```python
from build123d import *

# Parameters (mm, degrees)
F0_W            = 19
F0_H            = 19
F1_DEPTH        = 1
F2_W            = 17
F2_H            = 17
F3_DEPTH        = 4
F4_T            = 1
F4_T3_DEPTH     = 19
F4_T5_DEPTH     = 19
F6_DEPTH        = 2
F6_COPIES_COUNT = 4
F8_R            = 1
F9_SIZE         = 0.5


# Not quite as in the source:
# - a pattern or mirror of a feature is missing from the dataset's text; its kind, count and spacing are read off the source's solid
# - a shell that OpenCascade refuses in one call is made with other operations: the cavity is built on its own and cut out


with BuildPart() as f1:
    # F0 (on Top) → F1 (new body)
    with BuildSketch(Plane.XY):
        Rectangle(F0_W, F0_H)
    extrude(amount=F1_DEPTH)

    # F2 (on face) → F3 (join)
    with BuildSketch(Plane.XY.offset(1)):
        Rectangle(F2_W, F2_H)
    extrude(amount=F3_DEPTH)

    # F4: shell of thickness 1, made by hand


with BuildPart() as f4_core1:
    # F4_t2: copy of F1
    add(f1.part)

    # the walls: a layer under each face that stays
    f4_faces = [f4_core1.faces().sort_by_distance(p)[0] for p in [
        (0, -9.5, 0.5),
        (-9.5, 0, 0.5),
        (9.5, 0, 0.5),
        (0, 0, 0),
        (-8.8666666667, -8.8666666667, 1),
        (0, 9.5, 0.5),
        (8.5, 0, 3),
        (0, 8.5, 3),
        (-8.5, 0, 3),
        (0, -8.5, 3),
    ]]
    thicken(f4_faces, amount=-F4_T, mode=Mode.SUBTRACT)

    # F4_s4 → F4_t3 (cut)
    with BuildSketch(Plane.XZ.offset(-9.5)):
        Polygon((8.51, 1.01), (8.5, 0), (7.5, 0), (7.5, 1), align=None)
        Polygon((-8.51, 1.01), (-8.5, 0), (-7.5, 0), (-7.5, 1), align=None)
    extrude(amount=F4_T3_DEPTH, mode=Mode.SUBTRACT)

    # F4_s6 → F4_t5 (cut)
    with BuildSketch(Plane.YZ.offset(-9.5)):
        Polygon((8.51, 1.01), (8.5, 0), (7.5, 0), (7.5, 1), align=None)
        Polygon((-8.51, 1.01), (-8.5, 0), (-7.5, 0), (-7.5, 1), align=None)
    extrude(amount=F4_T5_DEPTH, mode=Mode.SUBTRACT)


with BuildPart() as f1_1:
    add(f1.part)

    # what is left inside the walls is the cavity
    f4_cavity = [f4_core1.part.solids().sort_by_distance(p)[0] for p in [
        (0, -2.5, 1.01),
    ]]
    add(f4_cavity, mode=Mode.SUBTRACT)

    # F5 (on face) → F6 (cut)
    with BuildSketch(Plane.XZ.offset(8.5)):
        with BuildLine():
            Line((5.5, 5), (-5.5, 5))
            ThreePointArc((-5.5, 5), (0, 2.8094750193), (5.5, 5))
        make_face()
    f6 = extrude(amount=-F6_DEPTH, mode=Mode.SUBTRACT)

    # F6_copies: F6 ×4 about axis
    f6_copies_axis = Axis((0, 0, 0), (0, 0, 1))
    for i in range(1, F6_COPIES_COUNT):
        add(f6.rotate(f6_copies_axis, i * 360 / F6_COPIES_COUNT), mode=Mode.SUBTRACT)

    # F8
    f8_edges = [f1_1.edges().sort_by_distance(p)[0] for p in [
        (-8.5, -8.5, 3),
        (-9.5, -9.5, 0.5),
        (8.5, -8.5, 3),
        (9.5, -9.5, 0.5),
        (8.5, 8.5, 3),
        (9.5, 9.5, 0.5),
        (-8.5, 8.5, 3),
        (-9.5, 9.5, 0.5),
    ]]
    fillet(f8_edges, radius=F8_R)

    # F9
    f9_edges = [f1_1.edges().sort_by_distance(p)[0] for p in [
        (6.5, 8.5, 5),
        (-6.5, 8.5, 5),
        (-8.5, 6.5, 5),
        (-8.5, -6.5, 5),
        (6.5, -8.5, 5),
        (8.5, -6.5, 5),
        (8.5, 6.5, 5),
        (8.207107, -8.207107, 5),
        (8.207107, 8.207107, 5),
        (-6.5, -8.5, 5),
        (-8.207107, -8.207107, 5),
        (-8.207107, 8.207107, 5),
    ]]
    chamfer(f9_edges, length=F9_SIZE)


solid = f1_1.part
```
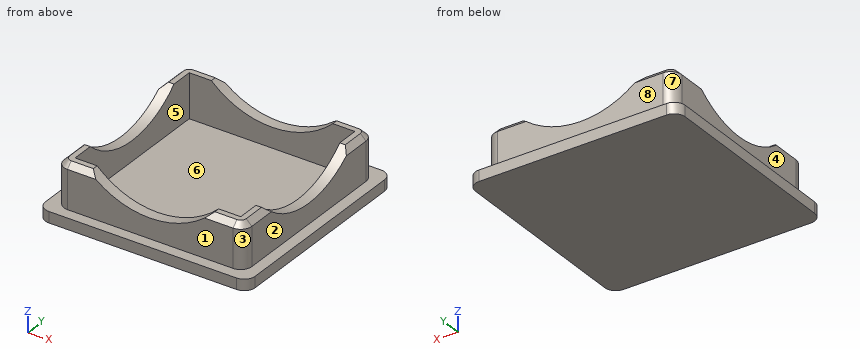
The model under review builds one solid part; all positions refer to its coordinate system, in mm. Face numbers are marked on the shaded views. A direction names the side the tool comes from. Round coordinates to 2 decimals unless told otherwise and drop trailing zeros. Loops run counter-clockwise (first coordinate to the right, second up) from the corner with the lowest first, then second, coordinate; pieces in that order, holes last.
1) Clearance check with flat-ended pins moving along their axes: P1, Ø1, axis at y = 1, z = 3.5, coming from the +X side; P2, Ø3, axis at x = 0.5, y = 1, coming from the -Z side; P3, Ø3, axis at x = -4, y = 3.5, coming from the +Z side; P4, Ø1.2, axis at y = -3, z = 2.5, coming from the +X side. State where each tip first meets the part, or that it passes through.
Values follow:
P1: passes through
P2: stops at z = 0
P3: stops at z = 1
P4: stops at x = 8.5
2) Consider section C-C on z = 3.95. State the section outline as (x, y) points.
Values follow:
outline: (-8.5, -7.5) arc R1 ccw to (-7.5, -8.5) - (-4.12, -8.5) - (-4.12, -7.5) - (-7.5, -7.5) - (-7.5, -4.12) - (-8.5, -4.12) - close; (-8.5, 4.12) - (-7.5, 4.12) - (-7.5, 7.5) - (-4.12, 7.5) - (-4.12, 8.5) - (-7.5, 8.5) arc R1 ccw to (-8.5, 7.5) - close; (4.12, -8.5) - (7.5, -8.5) arc R1 ccw to (8.5, -7.5) - (8.5, -4.12) - (7.5, -4.12) - (7.5, -7.5) - (4.12, -7.5) - close; (4.12, 7.5) - (7.5, 7.5) - (7.5, 4.12) - (8.5, 4.12) - (8.5, 7.5) arc R1 ccw to (7.5, 8.5) - (4.12, 8.5) - close
3) Consider section A-A on z = 1.5. State the section outline as (x, y) points.
Values follow:
outline: (-8.5, -7.5) arc R1 ccw to (-7.5, -8.5) - (7.5, -8.5) arc R1 ccw to (8.5, -7.5) - (8.5, 7.5) arc R1 ccw to (7.5, 8.5) - (-7.5, 8.5) arc R1 ccw to (-8.5, 7.5) - close; hole (-7.5, -7.5) - (7.5, -7.5) - (7.5, 7.5) - (-7.5, 7.5) - close
4) Wall thickness on line 1 along Y through (x, z) = (-6.5, 1.5); line 2 along Z through (x, y) = (3, 4): over which ranges is each line inside the solid? List them lowest first.
Values follow:
line 1: y = -8.5 to -7.5, 7.5 to 8.5
line 2: z = 0 to 1
5) Consider section B-B on x = 5.75. State the section outline as (y, z) points, then the cut area to 4 significant figures.
Values follow:
outline: (-9.5, 0) - (9.5, 0) - (9.5, 1) - (8.5, 1) - (8.5, 4.5) - (8, 5) - (7.5, 5) - (7.5, 1) - (-7.5, 1) - (-7.5, 5) - (-8, 5) - (-8.5, 4.5) - (-8.5, 1) - (-9.5, 1) - close
area: 26.75 mm2
6) Tool access review of the marked faces 1, 2, 3, 4 and 5: name each direction out of +Z, -Z, +X, -X, +Y, -Y from which nothing blocks a thin tool from reaching the whole face with its end or side.
Values follow:
face 1: +Z, +X, -X, -Y
face 2: +Z, +X, +Y, -Y
face 3: +Z, +X, -Y
face 4: +Z, -X, +Y, -Y
face 5: +Z
7) The part is to be moulded in two halves that separate along X. For the marked faces 6, 7 and 8, say which applies: pulls with the +X half, pulls with the -X half, needs draft (parallel to the pull), parting line crosses it, or undercut.
Values follow:
face 6: undercut
face 7: pulls with the -X half
face 8: needs draft
